Design review of the part built by this model. Coordinates are the model's own, in mm. Coordinates: 2 decimals unless noted, no trailing zeros. Write each loop counter-clockwise with the first axis right and the second up, starting at its lowest first coordinate (ties: lowest second). Pieces come first, ordered by that corner, then holes.
Q1. To check wall thickness, follow probe 1 along Y at (x, z) = (-375, -3); probe 2 along X at (y, z) = (128.5, -7.25). State the ranges of each line that lie inside material, in increasing order.
Q2. Add section B-B, the plane y = 105. Give the boundary of the cut face in (x, z), plus the area to 3 significant figures.
Q3. Clearance check with flat-ended pins moving along their axes: pin 1 Ø12 at (x, y) = (-141, 56.5) entering from -Z; pin 2 Ø3 at (x, z) = (-270.5, 3.5) entering from -Y; pin 3 Ø6 at (x, z) = (-112, -3.5) entering from +Y; pin 4 Ø6 at (y, z) = (30.5, -7.5) entering from -X. State where each tip first meets the part, or that it passes through.
Q4. Add section A-A, the plane z = -0.5. Give the boundary of the cut face in (x, y).
Q5. Add section C-C, the plane x = -193. Give the boundary of the cut face in (y, z), plus the area to 3 significant figures.
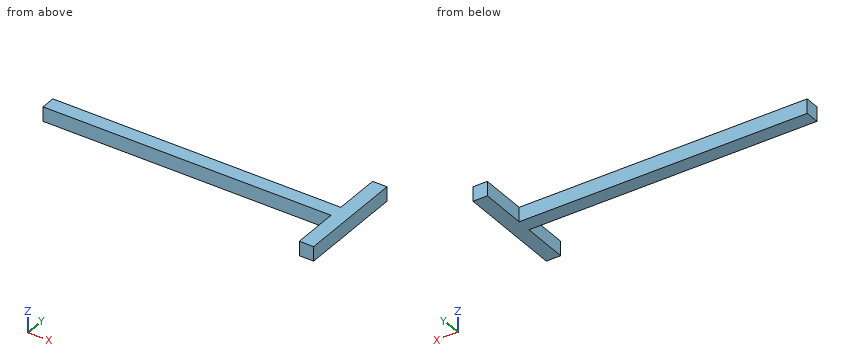
from build123d import *

# Parameters (mm, degrees)
SKETCH1_W           = 20
SKETCH1_H           = 20
BOSS_EXTRUDE1_DEPTH = 150
SKETCH2_W           = 20
SKETCH2_H           = 20
BOSS_EXTRUDE2_DEPTH = 400


with BuildPart() as part:
    # Sketch1 → Boss-Extrude1 (new body)
    with BuildSketch(Plane(origin=(0, 0, 0), x_dir=(1, 0, 0), z_dir=(0, 1, 0))):
        Rectangle(SKETCH1_W, SKETCH1_H)
    extrude(amount=BOSS_EXTRUDE1_DEPTH)

    # Sketch2 → Boss-Extrude2 (add)
    with BuildSketch(Plane.ZY.offset(10)):
        with Locations((0, 75)):
            Rectangle(SKETCH2_W, SKETCH2_H)
    extrude(amount=BOSS_EXTRUDE2_DEPTH)


solid = part.part
Here are the results:
1. probe 1: y = 65 to 85
1. probe 2: x = -10 to 10
2. outline: (-10, -10) - (10, -10) - (10, 10) - (-10, 10) - close
2. area: 400 mm2
3. pin 1: passes through
3. pin 2: stops at y = 65
3. pin 3: stops at y = 85
3. pin 4: stops at x = -10
4. outline: (-410, 65) - (-10, 65) - (-10, 0) - (10, 0) - (10, 150) - (-10, 150) - (-10, 85) - (-410, 85) - close
5. outline: (65, -10) - (85, -10) - (85, 10) - (65, 10) - close
5. area: 400 mm2
